Can you work these out from the drawing? Everything is in mm from the part's minimum corner. A direction names the side the tool comes from. Give positions to 0.01 mm unless a question says otherwise; leave off trailing zeros. Write each loop counter-clockwise with the first axis right and the second up, starting at its lowest first coordinate (ties: lowest second). Pieces come first, ordered by that corner, then holes. Notation, with made-up numbers: (47.25, 22.5) - (58.25, 22.5) arc R29 cw to (58.25, 61.5) - close; hole circle Ø9 at (39.5, -12.5). An arc over 180 degrees is marked (long way). Return JSON: item names as keys, results as strings. Group by question number.
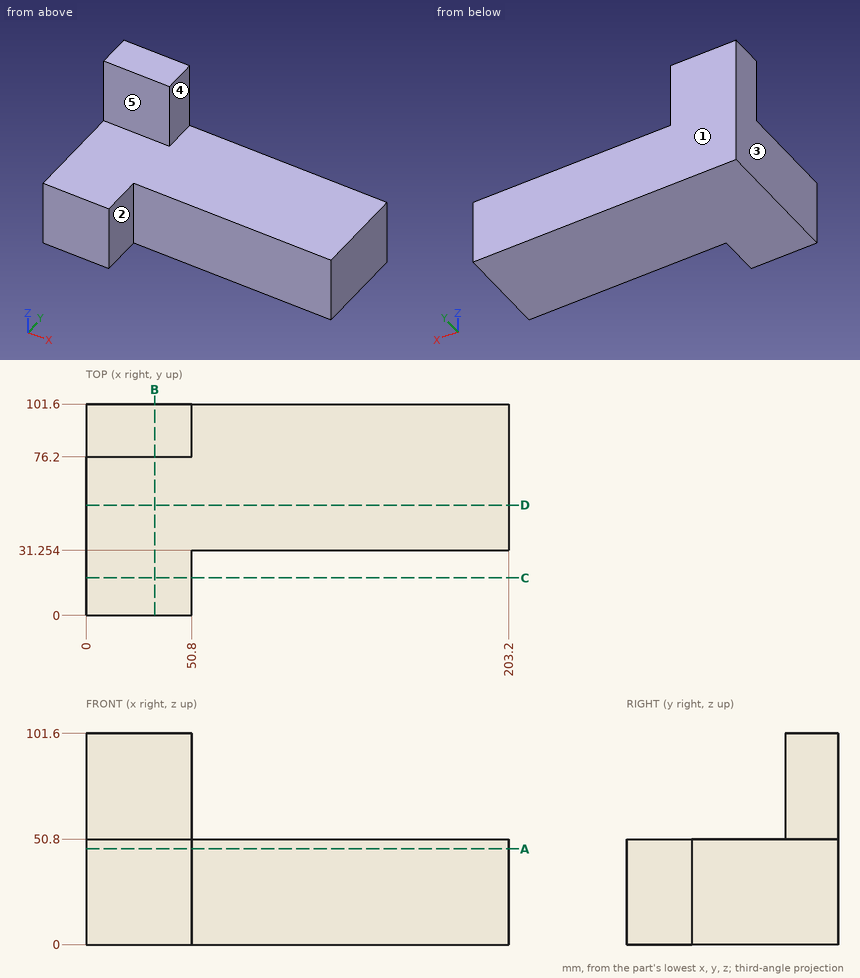
1) Imagine slicing it at D-D, the plane y = 53. Write out the boundary of the cut face in (x, z).
2) Imagine slicing it at C-C, the plane y = 18. Write out the boundary of the cut face in (x, z).
3) On a 3-axis mill with a long thin cutter (end or side, diameter ignored), from which of +Z, -Z, +X, -X, +Y, -Y can I reach the whole of each face in a straight line? I mean the marked faces 1, 2, 3, 4 and 5. Say none if no direction works.
4) Imagine slicing it at B-B, the plane x = 33. Write out the boundary of the cut face in (y, z).
5) I need wall thicknesses on line 1 along Z through (x, y) = (170, 57); line 2 along Y through (x, z) = (61.5, 15.5). Which ranges of each line are inside material? Lowest first, please.
6) Will these pins go through, and if not, where does the flat tip stop? pin 1 Ø1 at (x, z) = (106, 50) entering from -Y; pin 2 Ø6 at (y, z) = (86.5, 89.5) entering from +X; pin 3 Ø1.5 at (x, z) = (158, 53) entering from -Y.
7) Imagine slicing it at A-A, the plane z = 46. Write out the boundary of the cut face in (x, y), and give its area (3 significant figures).
Resolved:
{
 "1": {"outline": "(0, 0) - (203.2, 0) - (203.2, 50.8) - (0, 50.8) - close"},
 "2": {"outline": "(0, 0) - (50.8, 0) - (50.8, 50.8) - (0, 50.8) - close"},
 "3": {"face 1": "+Z, -Z, +X, -X, +Y", "face 2": "+Z, -Z, +X, -Y", "face 3": "+Z, -Z, -X, +Y, -Y", "face 4": "+Z, +X, +Y, -Y", "face 5": "+Z, +X, -X, -Y"},
 "4": {"outline": "(0, 0) - (101.6, 0) - (101.6, 101.6) - (76.2, 101.6) - (76.2, 50.8) - (0, 50.8) - close"},
 "5": {"line 1": "0 to 50.8", "line 2": "31.25 to 101.6"},
 "6": {"pin 1": "y = 31.25", "pin 2": "x = 50.8", "pin 3": "through"},
 "7": {"outline": "(0, 0) - (50.8, 0) - (50.8, 31.25) - (203.2, 31.25) - (203.2, 101.6) - (0, 101.6) - close", "area": "15,900 mm^2"}
}
